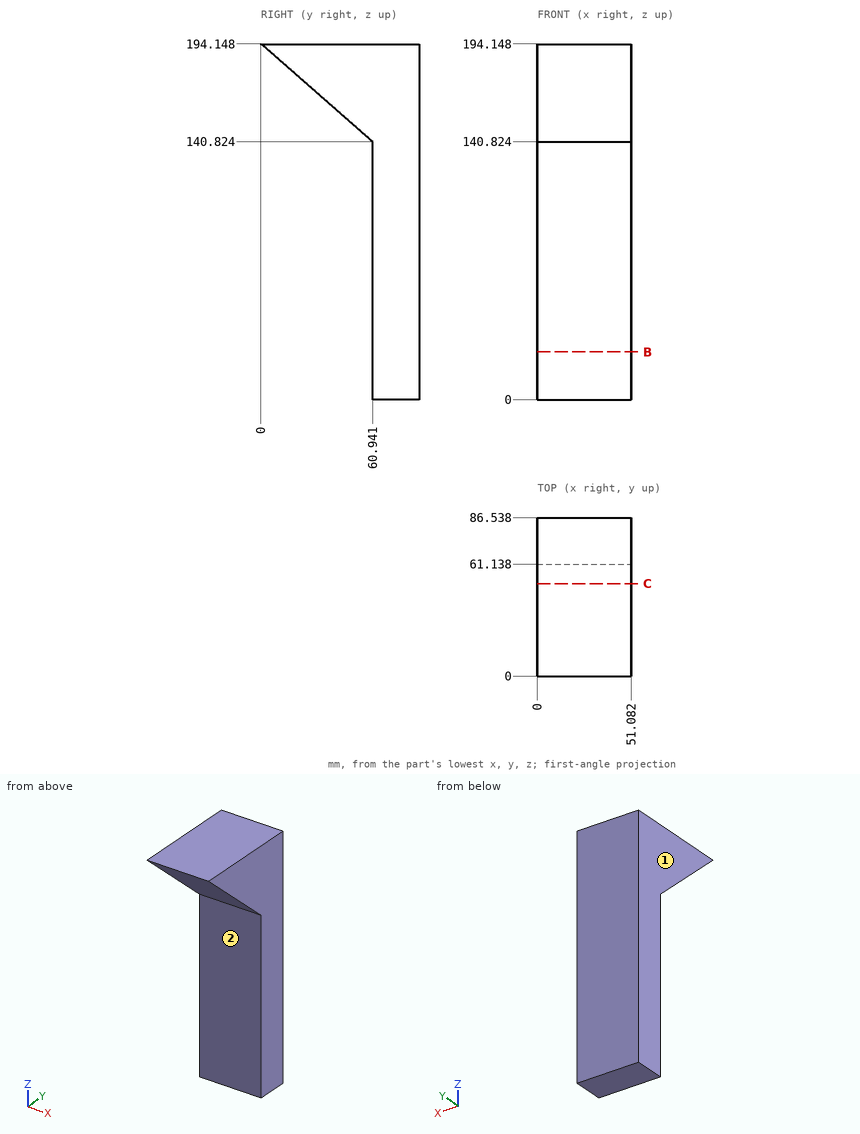
Print and shaded views of the part. All mm, measured from the part's lowest x, y and z. A direction names the side the tool comes from. Round coordinates to 2 decimals unless told otherwise and drop trailing zeros. Write each loop counter-clockwise with the first axis right and the second up, starting at its lowest first coordinate (ties: lowest second). Pieces come first, ordered by that corner, then holes. Notation, with made-up numbers: M -15.75,23.25 L -1.75,23.25 A11 ccw -1.75,29.25 Z; hole C -28.5,18 d11. An arc over 180 degrees is marked long. Use a Markdown table: item, result. Add a question column.
1. Flat gauge pins, fed straight in: P1, Ø10, axis at x = 39, z = 82, coming from the -Y side; P2, Ø8, axis at x = 9, y = 75.5, coming from the -Z side; P3, Ø8, axis at x = 46, y = 25.5, coming from the -Z side (1 decimal). Where does each tip first touch, or does it go through?
2. Drill centre lines: probe 1 along Y at (x, z) = (17.5, 29.5); probe 2 along Z at (x, y) = (27.5, 16); probe 3 along Y at (x, z) = (43.5, 182) (1 decimal). Where is each one in solid material? Low to high.
3. Slice it at C-C on y = 50.5. Give the cut face in (x, z), then the cut area to 3 significant figures.
4. 3-axis set-ups, long thin cutter, end or side, ignore diameter. For the marked faces 1 and 2: which of +Z, -Z, +X, -X, +Y, -Y reach the whole face in a straight line?
5. Slice it at B-B on z = 26. Give the cut face in (x, y), then the cut area to 3 significant figures.
Reply:
| question | item | result |
|---|---|---|
| 1 | P1 | stops at y = 61.14 |
| 1 | P2 | stops at z = 0 |
| 1 | P3 | stops at z = 168.3 |
| 2 | probe 1 | y = 61.14 to 86.54 |
| 2 | probe 2 | z = 180.15 to 194.15 |
| 2 | probe 3 | y = 13.9 to 86.5 |
| 3 | outline | M 0,149.96 L 51.08,149.96 L 51.08,194.15 L 0,194.15 Z |
| 3 | area | 2,260 mm^2 |
| 4 | face 1 | +Z, -Z, -X, +Y, -Y |
| 4 | face 2 | -Z, +X, -X, -Y |
| 5 | outline | M 0,61.14 L 51.08,61.14 L 51.08,86.54 L 0,86.54 Z |
| 5 | area | 1,300 mm^2 |
